Could you check a few things on this drawing? It's one solid part, dimensions in mm from its lowest x, y, z. A direction names the side the tool comes from. Give positions to 0.01 mm unless a question says otherwise; leave off trailing zeros. Order: outer loops, then holes, each group sorted by start corner. A loop starts at its lowest first (then second) coordinate and runs counter-clockwise, first axis right, second up. Notation, with made-up numbers: (38, -35) -> (66, -35) arc R16 ccw to (66, -27) -> close; hole circle Ø5 at (17, 69.25). An arc over 180 degrees is marked (long way). Answer as a JSON object with one key per item and string values.
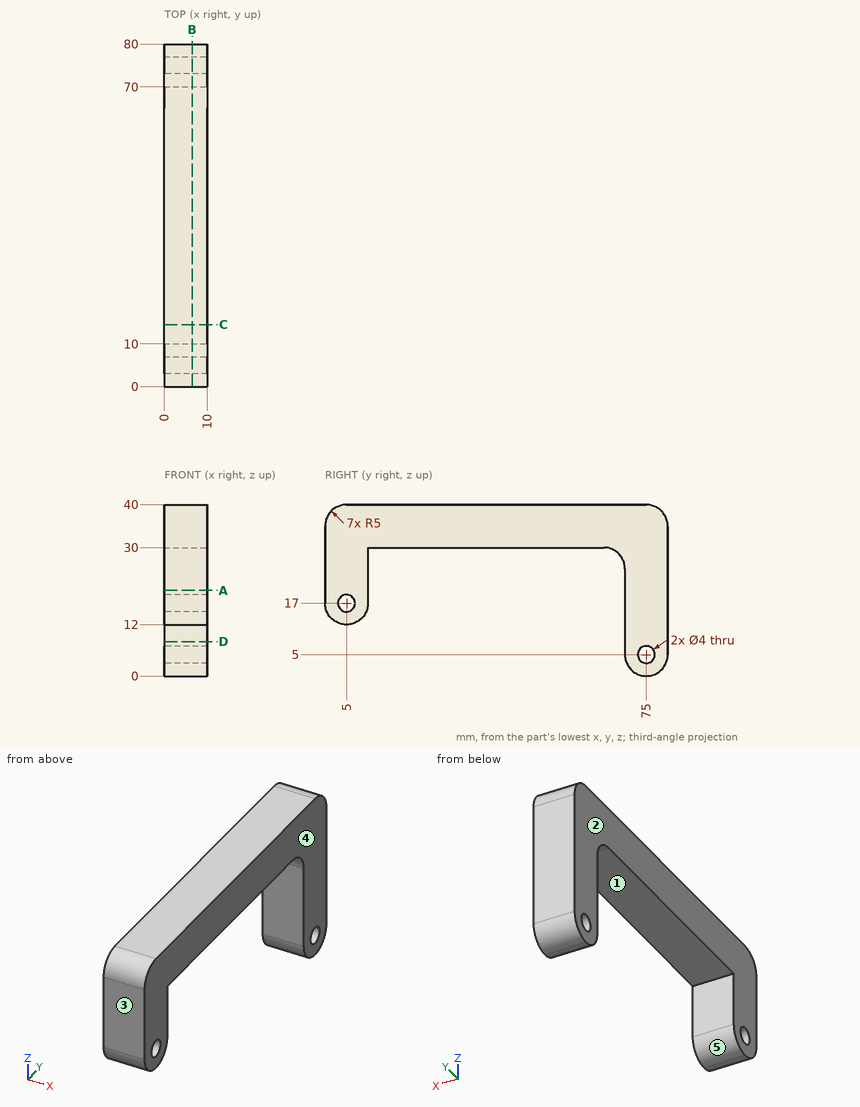
1. If we section it at B-B on x = 6.5: Count the separate pieces of the cut face and the enclosed holes in it, then the cut area to 3 significant figures.
Worked answers:
{"separate pieces": "1", "enclosed holes": "2", "area": "1,230 mm²"}
2. For the marked faces 1 and 2, which set-ups out of +Z, -Z, +X, -X, +Y, -Y let a thin tool reach every point of the face, with its end or its side?
Worked answers:
{"face 1": "-Z, +X, -X", "face 2": "+Z, -Z, -X, +Y, -Y"}
3. If we mould it in two halves opening along Y, with no side actions, what happens to the marked faces 3, 4 and 5? For each: +Y half, -Y half, draft (parallel to the pull), parting line (faces both ways), or undercut.
Worked answers:
{"face 3": "-Y half", "face 4": "draft", "face 5": "undercut"}
4. Will these pins go through, and if not, where does the flat tip stop? pin 1 Ø2 at (x, y) = (5.5, 41) entering from -Z; pin 2 Ø4 at (x, z) = (6, 11) entering from -Y; pin 3 Ø1.5 at (x, y) = (3.5, 65.5) entering from -Z.
Worked answers:
{"pin 1": "z = 30", "pin 2": "y = 2", "pin 3": "z = 29.84"}
5. If we section it at A-A on z = 20: Please give me the cut outline in (x, y), then the cut area to 3 significant figures.
Worked answers:
{"outline": "(0, 0) -> (10, 0) -> (10, 10) -> (0, 10) -> close; (0, 70) -> (10, 70) -> (10, 80) -> (0, 80) -> close", "area": "200 mm²"}
6. If we section it at D-D on z = 8: Please give me the cut outline in (x, y).
Worked answers:
{"outline": "(0, 70) -> (10, 70) -> (10, 80) -> (0, 80) -> close"}
7. Please list where these lines run through material, in increasing order: L1, parallel to Z at x = 7, y = 5; L2, parallel to Z at x = 6.5, y = 75; L3, parallel to Y at x = 5.5, z = 8.
Worked answers:
{"L1": "12 to 15, 19 to 40", "L2": "0 to 3, 7 to 40", "L3": "70 to 80"}
8. If we section it at C-C on y = 14.5: Please give me the cut outline in (x, z).
Worked answers:
{"outline": "(0, 30) -> (10, 30) -> (10, 40) -> (0, 40) -> close"}
